from build123d import *

# Parameters (mm, degrees)
SKETCH_1_W      = 5.999999173
SKETCH_1_H      = 10.999998182
SKETCH_1_W_2    = 4.00000019
SKETCH_1_H_2    = 8.999999777
SKETCH_1_H_3    = 9.000000708
SKETCH_1_W_3    = 4.000000656
EXTRUDE_1_DEPTH = 3


with BuildPart() as part:
    # 草图1 → 凸台-拉伸1 (new body)
    with BuildSketch(Plane.XY):
        with BuildLine():
            Line((9.999999777, 25.999999166), (9.999999777, 33.000000149))
            Line((9.999999777, 33.000000149), (7.000000216, 33.000000149))
            Line((7.000000216, 33.000000149), (7.000000216, 30.499998808))
            ThreePointArc((7.000000216, 30.499998808), (7.353551416, 29.64644555), (6.500000134, 30.00000152))
            Line((6.500000134, 30.00000152), (3.500000108, 30.00000152))
            ThreePointArc((3.500000108, 30.00000152), (2.646448658, 29.646445383), (3.000000026, 30.499998808))
            Line((3.000000026, 30.499998808), (3.000000026, 33.000000149))
            Line((3.000000026, 33.000000149), (0, 33.000000149))
            Line((0, 33.000000149), (0, 0))
            Line((0, 0), (3.000000026, 0))
            Line((3.000000026, 0), (3.000000026, 2.499999944))
            ThreePointArc((3.000000026, 2.499999944), (2.64644665, 3.353553403), (3.500000108, 3.000000026))
            Line((3.500000108, 3.000000026), (6.500000134, 3.000000026))
            ThreePointArc((6.500000134, 3.000000026), (7.353553425, 3.353553235), (7.000000216, 2.499999944))
            Line((7.000000216, 2.499999944), (7.000000216, 0))
            Line((7.000000216, 0), (9.999999777, 0))
            Line((9.999999777, 0), (9.999999777, 7.000000983))
            Line((9.999999777, 7.000000983), (16.00000076, 7.000000983))
            Line((16.00000076, 7.000000983), (16.00000076, 0))
            Line((16.00000076, 0), (18.999999389, 0))
            Line((18.999999389, 0), (18.999999389, 2.499999944))
            ThreePointArc((18.999999389, 2.499999944), (18.646447034, 3.353553971), (19.500000402, 3.000000026))
            Line((19.500000402, 3.000000026), (22.500000894, 3.000000026))
            ThreePointArc((22.500000894, 3.000000026), (23.353554637, 3.353553028), (23.000000045, 2.499999944))
            Line((23.000000045, 2.499999944), (23.000000045, 0))
            Line((23.000000045, 0), (26.000000536, 0))
            Line((26.000000536, 0), (26.000000536, 33.000000149))
            Line((26.000000536, 33.000000149), (23.000000045, 33.000000149))
            Line((23.000000045, 33.000000149), (23.000000045, 30.499998808))
            ThreePointArc((23.000000045, 30.499998808), (23.353552628, 29.646445757), (22.500000894, 30.00000152))
            Line((22.500000894, 30.00000152), (19.500000402, 30.00000152))
            ThreePointArc((19.500000402, 30.00000152), (18.646449043, 29.646444814), (18.999999389, 30.499998808))
            Line((18.999999389, 30.499998808), (18.999999389, 33.000000149))
            Line((18.999999389, 33.000000149), (16.00000076, 33.000000149))
            Line((16.00000076, 33.000000149), (16.00000076, 25.999999166))
            Line((16.00000076, 25.999999166), (9.999999777, 25.999999166))
        make_face()
        with Locations((12.999999802, 16.500000075)):
            Rectangle(SKETCH_1_W, SKETCH_1_H, mode=Mode.SUBTRACT)
        with Locations((5.000000121, 22.499999278)):
            Rectangle(SKETCH_1_W_2, SKETCH_1_H_2, mode=Mode.SUBTRACT)
        with Locations((5.000000121, 10.500000406)):
            Rectangle(SKETCH_1_W_2, SKETCH_1_H_3, mode=Mode.SUBTRACT)
        with Locations((20.999999717, 10.500000406)):
            Rectangle(SKETCH_1_W_3, SKETCH_1_H_3, mode=Mode.SUBTRACT)
        with Locations((20.999999717, 22.499999278)):
            Rectangle(SKETCH_1_W_3, SKETCH_1_H_2, mode=Mode.SUBTRACT)
    extrude(amount=EXTRUDE_1_DEPTH)


solid = part.part
Here's how the part is built. I have some questions about the finished solid (model axes, mm). A direction names the side the tool comes from. Give positions to 0.01 mm unless a question says otherwise; leave off trailing zeros. Order: outer loops, then holes, each group sorted by start corner. A loop starts at its lowest first (then second) coordinate and runs counter-clockwise, first axis right, second up. Notation, with made-up numbers: (-24, 4) -> (19, 4) arc R22 cw to (19, 42) -> close; hole circle Ø3 at (19, 9.5). An arc over 180 degrees is marked (long way). One line per item, written item: value. Start each with the question number.
1. Imagine slicing it at A-A, the plane x = 14.75. List the corners of the cut face in (y, z) for me.
2. For faces 1 (the face through (13, 26, 1)), 2 (the face through (10, 3, 1)), 3 (the face through (21, 15, 1)), which set-ups out of +Z, -Z, +X, -X, +Y, -Y let a thin tool reach every point of the face, with its end or its side?
3. Imagine slicing it at B-B, the plane y = 10.5. List the corners of the cut face in (x, z) for me, plus the area to 3 significant figures.
4. I need wall thicknesses on probe 1 along X at (y, z) = (12, 1.6); probe 2 along Y at (x, z) = (21.25, 1.15); probe 3 along X at (y, z) = (9.5, 1.15). Which ranges of each line are inside material? Lowest first, please. Write a range as from..to.
5. Will these pins go through, and if not, where does the flat tip stop? pin 1 Ø1 at (x, z) = (15, 2.5) entering from -Y; pin 2 Ø3 at (x, y) = (10.5, 5) entering from +Z; pin 3 Ø1.5 at (x, z) = (20.5, 1) entering from -Y; pin 4 Ø0.9 at (x, z) = (21, 2) entering from +Y.
6. We'd pull the mould along X, two halves only. Please class faces 4 (the face through (13, 11, 1)), 5 (the face through (24, 0, 1)): released by +X, released by -X, zero draft, split by the parting line, or undercut.
7. Imagine slicing it at C-C, the plane z = 0.5. Count the separate pieces of the cut face and the enclosed holes in it, plus the area to 3 significant figures.
Values follow:
1. outline: (7, 0) -> (11, 0) -> (11, 3) -> (7, 3) -> close; (22, 0) -> (26, 0) -> (26, 3) -> (22, 3) -> close
2. face 1: +Z, -Z, +Y
2. face 2: +Z, -Z, -Y
2. face 3: +Z, -Z
3. outline: (0, 0) -> (3, 0) -> (3, 3) -> (0, 3) -> close; (7, 0) -> (19, 0) -> (19, 3) -> (7, 3) -> close; (23, 0) -> (26, 0) -> (26, 3) -> (23, 3) -> close
3. area: 54.0 mm2
4. probe 1: x = 0..3, 7..10, 16..19, 23..26
4. probe 2: y = 3..6, 15..18, 27..30
4. probe 3: x = 0..3, 7..19, 23..26
5. pin 1: stops at y = 7
5. pin 2: stops at z = 3
5. pin 3: stops at y = 3
5. pin 4: stops at y = 30
6. face 4: undercut
6. face 5: zero draft
7. separate pieces: 1
7. enclosed holes: 5
7. area: 511 mm2
